Model file for the job. Use its own axes, mm. Face numbers are marked on the shaded views. A direction names the side the tool comes from. Coordinates: 2 decimals unless noted, no trailing zeros. Write each loop counter-clockwise with the first axis right and the second up, starting at its lowest first coordinate (ties: lowest second). Pieces come first, ordered by that corner, then holes. Notation, with made-up numbers: (-3.75, 78.25) -> (4.25, 78.25) arc R12 ccw to (4.25, 92.25) -> close; hole circle Ø10 at (51, 5.5). An arc over 180 degrees is marked (long way). Write item = value, one per line. Start each with the question number.
from build123d import *

# Parameters (mm, degrees)
F1_DEPTH      = 76.2
F2_DEPTH      = 25.4
F2_DEPTH_BACK = 101.6
F3_R          = 7.7865248509
F4_DEPTH      = 101.6
F5_R          = 7.747
F6_DEPTH      = 101.6


with BuildPart() as f1:
    # F0 (on Front) → F1 (new body)
    with BuildSketch(Plane.XZ):
        with BuildLine():
            Line((-50.9560853243, -35.3116765618), (50.9560853243, -35.3116765618))
            Line((50.9560853243, -35.3116765618), (50.9560853243, 35.3116765618))
            Line((50.9560853243, 35.3116765618), (35.56, 35.3116765618))
            ThreePointArc((35.56, 35.3116765618), (0, 11.5130765942), (-35.56, 35.3116765618))
            Line((-35.56, 35.3116765618), (-50.9560853243, 35.3116765618))
            Line((-50.9560853243, 35.3116765618), (-50.9560853243, -35.3116765618))
        make_face()
    extrude(amount=F1_DEPTH)

    # F0 (on Front) → F2 (join, two sides)
    with BuildSketch(Plane.XZ) as f2_sk:
        with BuildLine():
            ThreePointArc((-35.56, 35.3116765618), (0, 11.5130765942), (35.56, 35.3116765618))
            Line((35.56, 35.3116765618), (22.6471517235, 35.3116765618))
            ThreePointArc((22.6471517235, 35.3116765618), (0, 18.5039060672), (-22.6471517235, 35.3116765618))
            Line((-22.6471517235, 35.3116765618), (-35.56, 35.3116765618))
        make_face()
    extrude(amount=-F2_DEPTH)
    extrude(f2_sk.sketch, amount=F2_DEPTH_BACK)

    # F3 (on face) → F4 (cut)
    with BuildSketch(Plane.XY.offset(35.3116765618)):
        with Locations((35.56, -38.1)):
            Circle(F3_R)
    extrude(amount=-F4_DEPTH, mode=Mode.SUBTRACT)

    # F5 (on face) → F6 (cut)
    with BuildSketch(Plane.XY.offset(35.3116765618)):
        with Locations((-35.56, -38.1)):
            Circle(F5_R)
    extrude(amount=-F6_DEPTH, mode=Mode.SUBTRACT)


solid = f1.part
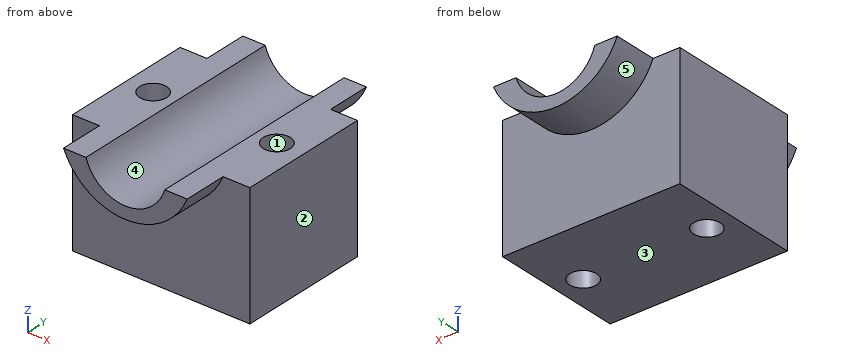
(1) Saw through at C-C (z = -28). Give the cut face in (x, y), then the cut area to 3 significant figures.
(2) Saw through at B-B (z = 26.5). Give the cut face in (x, y), then the cut area to 3 significant figures.
(3) Drill centre lines: line 1 along X through (y, z) = (-38, -14); line 2 along Y through (x, z) = (-35.56, -15.5); line 3 along Y through (x, z) = (35, 0). Where is each one in solid material? Low to high.
(4) Saw through at D-D (x = -32). Give the cut face in (y, z), then the cut area to 3 significant figures.
(5) 3-axis set-ups, long thin cutter, end or side, ignore diameter. For the marked faces 4 and 5: which of +Z, -Z, +X, -X, +Y, -Y reach the whole face in a straight line?
(6) Saw through at A-A (y = -38.1). Give the cut face in (x, z).
(7) Mould opens along X. For the marked faces 1, 2 and 3 say: released by +X, released by -X, zero draft, split by the parting line, or undercut.
(8) Drop flat-ended pins along their axis: pin 1 Ø4 at (x, y) = (-16.5, -74) entering from +Z; pin 2 Ø21 at (x, z) = (20.5, -6) entering from +Y; pin 3 Ø4 at (x, z) = (-14, 5.5) entering from -Y; pin 4 Ø14 at (x, y) = (-35.56, -38.1) entering from +Z. Give the stop position or say it passes through.
Returned:
q1.outline = (-50.96, -76.2) -> (50.96, -76.2) -> (50.96, 0) -> (-50.96, 0) -> close; hole circle Ø15.49 at (-35.56, -38.1); hole circle Ø15.57 at (35.56, -38.1)
q1.area = 7,390 mm2
q2.outline = (-50.96, -76.2) -> (-30.47, -76.2) -> (-30.47, -101.6) -> (-17.73, -101.6) -> (-17.73, 25.4) -> (-30.47, 25.4) -> (-30.47, 0) -> (-50.96, 0) -> close; (17.73, -101.6) -> (30.47, -101.6) -> (30.47, -76.2) -> (50.96, -76.2) -> (50.96, 0) -> (30.47, 0) -> (30.47, 25.4) -> (17.73, 25.4) -> close; hole circle Ø15.49 at (-35.56, -38.1); hole circle Ø15.57 at (35.56, -38.1)
q2.area = 5,980 mm2
q3.line_1 = -50.96 to -43.31, -27.81 to 27.77, 43.35 to 50.96
q3.line_2 = -76.2 to -45.85, -30.35 to 0
q3.line_3 = -76.2 to -45.87, -30.33 to 0
q4.outline = (-101.6, 28.63) -> (-76.2, 28.63) -> (-76.2, -35.31) -> (-44.98, -35.31) -> (-44.98, 35.31) -> (-101.6, 35.31) -> close; (-31.22, -35.31) -> (0, -35.31) -> (0, 28.63) -> (25.4, 28.63) -> (25.4, 35.31) -> (-31.22, 35.31) -> close
q4.area = 4,750 mm2
q5.face_4 = +Z, +Y, -Y
q5.face_5 = -Z, +Y
q6.outline = (-50.96, -35.31) -> (-43.31, -35.31) -> (-43.31, 35.31) -> (-50.96, 35.31) -> close; (-27.81, -35.31) -> (27.77, -35.31) -> (27.77, 35.31) -> (22.65, 35.31) arc R23.66 cw to (-22.65, 35.31) -> (-27.81, 35.31) -> close; (43.35, -35.31) -> (50.96, -35.31) -> (50.96, 35.31) -> (43.35, 35.31) -> close
q7.face_1 = undercut
q7.face_2 = released by +X
q7.face_3 = zero draft
q8.pin_1 = 27.41
q8.pin_2 = 0
q8.pin_3 = -76.2
q8.pin_4 = through
